Could you check a few things on this model? Use its own coordinates, in mm. Coordinates: 2 decimals unless noted, no trailing zeros. Write each loop counter-clockwise with the first axis right and the second up, starting at its lowest first coordinate (ties: lowest second). Pieces come first, ordered by that corner, then holes. Notation, with made-up numbers: M 59,20 L 80,20 A26 cw 80,45 Z; hole C -8.5,9 d1. An arc over 180 degrees is marked long. Answer as CSV lines item,"result". Start each with the question number.
Item 1: We'd pull the mould along Z, two halves only. Please class faces 1 (the flat face through (5, 6, 0)), 2 (the flat face through (5.02, 5.47, 5.87)), 3 (the flat face through (5, 0, 44)): +Z half, -Z half, draft (parallel to the pull), parting line (faces both ways), or undercut.
Item 2: If I drill on line 1 along Z through (x, y) = (6.5, 7); line 2 along Z through (x, y) = (5.25, 0.75); line 3 along Y through (x, z) = (7.75, 20), over which ranges is the centre line in solid material (lowest first)? Write a range as [from, to].
Item 3: Suppose I cut it at B-B, the plane z = 57. Write out the boundary of the cut face in (x, y).
Item 4: Suppose I cut it at A-A, the plane x = 5. Write out the boundary of the cut face in (y, z).
Item 5: I'm going to push flat-ended pins straight in: P1, Ø4, axis at y = 6, z = 7, coming from the -X side; P2, Ø2, axis at x = 3, y = 4.5, coming from the -Z side; P3, Ø3, axis at y = 0, z = 0, coming from the +X side. Where does each tip first touch, or does it pass through?
Autodesk Inventor part; units mm, degrees
ref_plane "Work Plane1" through (5, 0, 85) normal (1, 0, 0) x (0, 0, -1)
ref_plane "YZ Plane" through (0, 0, 0) normal (1, 0, 0) x (0, 1, 0)
ref_plane "XZ Plane" through (0, 0, 0) normal (0, 1, 0) x (-1, 0, 0)
sketch "Base" plane through (0, 0, 0) normal (0, 1, 0) x (-1, 0, 0)
  line L0 (0, 0) -> (-10, 0)
  line L1 (-10, 0) -> (-10, 85)
  line L2 (-10, 85) -> (0, 85)
  line L3 (0, 85) -> (0, 0)
  dimension "KeyWidth" = 10
  dimension "KeyLength" = 85
extrude "Main Body" add sketch "Base" along normal blind 10
sketch "Hinge Sketch" plane through (10, 0, 85) normal (1, 0, 0) x (0, 0, -1)
  circle A0 centre (85, 0) radius 1.7
  circle A1 centre (85, 0) radius 2.7
  dimension "d10" = 3.4
  dimension "d11" = 1
extrude "Hinge Surround" add sketch "Hinge Sketch" against normal up to surface (10 mm away)
extrude "Hinge Hole" cut sketch "Hinge Sketch" against normal up to next contours A0
ref_plane "Work Plane1" through (5, 0, 85) normal (1, 0, 0) x (0, 0, -1)
sketch "Sweep Path" plane through (5, 0, 85) normal (1, 0, 0) x (0, 0, -1)
  arc A0 (79.1465, 5.4531) -> (77, 0) centre (85, 0) ccw
  line L0 (0, 0) -> (82.3, 0) construction
  dimension "SweepAngle" = 42.972
  dimension "SweepRadius" = 8
sketch "Sweep Profile" plane through (0, 0, 0) normal (0, -1, 0) x (1, 0, 0)
  circle A0 centre (5, 8) radius 1.5
  point P0 (0, 0)
  dimension "RingThickness" = 3
sweep "Sweep2" cut profiles "Sweep Profile" path "Sweep Path"
equation "\"KeyWidth\" = MaxWidth"
equation "\"SweepArcLength\" = 6"
properties part number "Key0"
Ans:
1,face 1,"-Z half"
1,face 2,"undercut"
1,face 3,"draft"
2,line 1,"z = [0, 85]"
2,line 2,"z = [-2.59, -1.53], [1.53, 6.48], [9.45, 85]"
2,line 3,"y = [0, 10]"
3,outline,"M 0,0 L 10,0 L 10,10 L 0,10 Z"
4,outline,"M 0,2.7 A2.7 ccw long 2.7,0 L 10,0 L 10,85 L 0,85 L 0,9.5 A9.5 cw 6.48,6.95 L 4.43,4.76 A6.5 ccw 0,6.5 Z; hole C 0,0 d3.4"
5,P1,"stops at x = 0"
5,P2,"stops at z = 0"
5,P3,"passes through"
